Design review of the part shown in the three views and the two pictorial views. Dimensions are in mm from the part's minimum x, y and z. Give positions to 0.01 mm unless a question says otherwise; leave off trailing zeros. Loops run counter-clockwise (first coordinate to the right, second up) from the corner with the lowest first, then second, coordinate; pieces in that order, holes last. Notation, with made-up numbers: M 64.25,78.25 L 99.25,78.25 A21 ccw 99.25,94.25 Z; hole C 29.5,-19.5 d8. An arc over 180 degrees is marked long. Return JSON: item names as keys, results as strings. Group by question number.
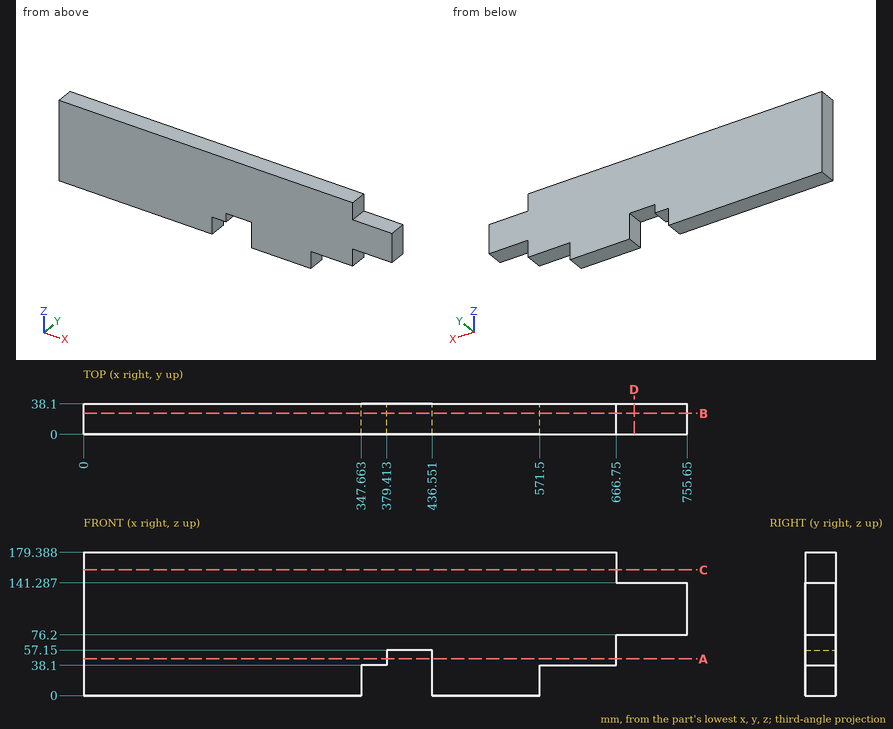
(1) For pin 1 (19 mm diameter, centred on y = 18.5, z = 20, fed in from +X); pin 2 (11.5 mm diameter, centred on y = 12.5, z = 160, fed in from +X); pin 3 (1.5 mm diameter, centred on x = 433.5, y = 10.5, fed in from -Z), all flat-tipped, find the tip position at first contact; note any pin that passes through.
(2) Add section A-A (z = 46). Write out the cut boundary in (x, y), and give its area (3 significant figures).
(3) Add section D-D (x = 689.5). Write out the cut boundary in (y, z), and give its area (3 significant figures).
(4) For probe 1 along X at (y, z) = (18.5, 21); probe 2 along Z at (x, y) = (637, 17); probe 3 along Z at (x, y) = (707, 16.5), list the stretches that pass through material, from the lowest coordinate up.
(5) Add section C-C (z = 157.5). Write out the cut boundary in (x, y).
(6) Add section B-B (y = 26.5). Write out the cut boundary in (x, z), and give its area (3 significant figures).
Verdict:
{
 "1": {"pin 1": "stops at x = 571.5", "pin 2": "stops at x = 666.75", "pin 3": "stops at z = 57.15"},
 "2": {"outline": "M 0,0 L 379.41,0 L 379.41,38.1 L 0,38.1 Z; M 436.55,0 L 666.75,0 L 666.75,38.1 L 436.55,38.1 Z", "area": "23,200 mm²"},
 "3": {"outline": "M 0,76.2 L 38.1,76.2 L 38.1,141.29 L 0,141.29 Z", "area": "2,480 mm²"},
 "4": {"probe 1": "x = 0 to 347.66, 436.55 to 571.5", "probe 2": "z = 38.1 to 179.39", "probe 3": "z = 76.2 to 141.29"},
 "5": {"outline": "M 0,0 L 666.75,0 L 666.75,38.1 L 0,38.1 Z"},
 "6": {"outline": "M 0,0 L 347.66,0 L 347.66,38.1 L 379.41,38.1 L 379.41,57.15 L 436.55,57.15 L 436.55,0 L 571.5,0 L 571.5,38.1 L 666.75,38.1 L 666.75,76.2 L 755.65,76.2 L 755.65,141.29 L 666.75,141.29 L 666.75,179.39 L 0,179.39 Z", "area": "117,000 mm²"}
}
